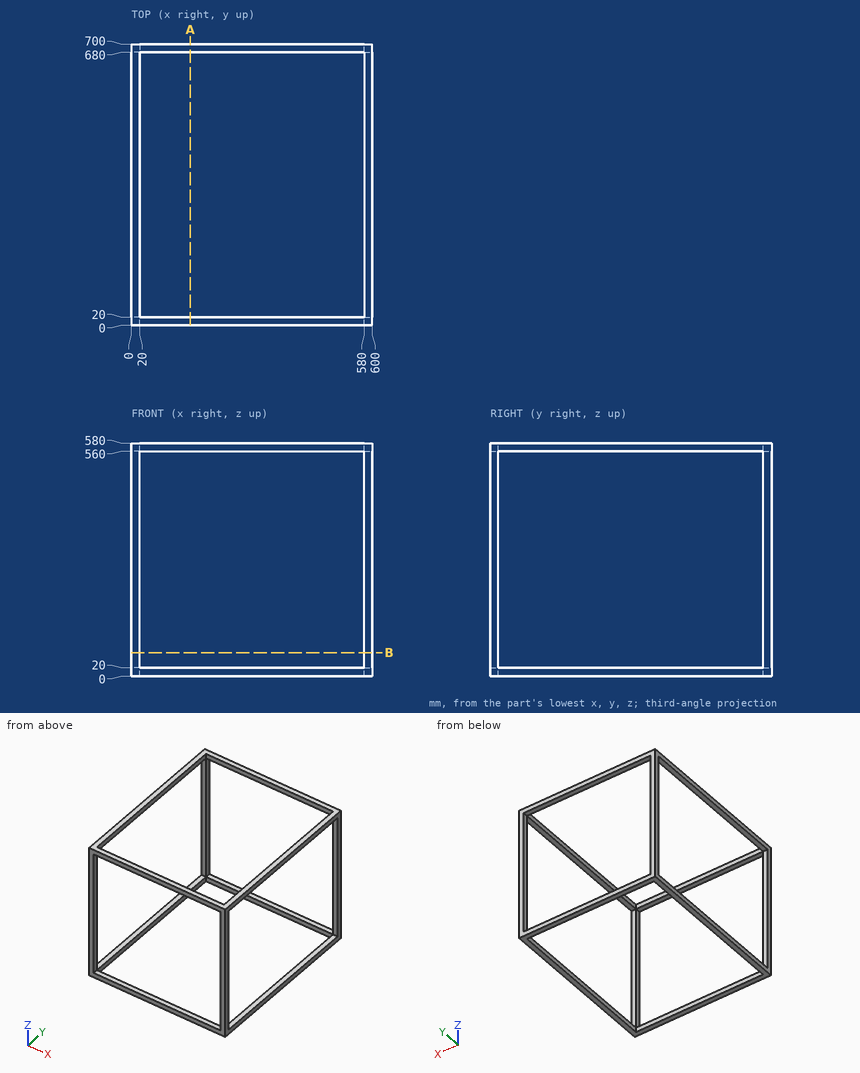
Source: three-view drawing plus pictorial views. Frame: mm from the lowest corner of the part. Give positions to 0.01 mm unless a question says otherwise; leave off trailing zeros. Write each loop counter-clockwise with the first axis right and the second up, starting at its lowest first coordinate (ties: lowest second). Pieces come first, ordered by that corner, then holes. Notation, with made-up numbers: (-23.75, 30) -> (22.25, 30) arc R34 cw to (22.25, 60) -> close; hole circle Ø3 at (87.5, -19.75). An arc over 180 degrees is marked (long way). Write item = value, one per line.
Q1. Cut plane A-A on x = 146.5. Return loops of the section in (y, z), then the cut area to 3 significant figures.
Here are the results:
outline = (0, 0) -> (20, 0) -> (20, 20) -> (0, 20) -> close; (0, 560) -> (20, 560) -> (20, 580) -> (0, 580) -> close; (680, 0) -> (700, 0) -> (700, 20) -> (680, 20) -> close; (680, 560) -> (700, 560) -> (700, 580) -> (680, 580) -> close
area = 1,600 mm²
Q2. Cut plane B-B on z = 58.5. Return loops of the section in (x, y), then the cut area to 3 significant figures.
Here are the results:
outline = (0, 0) -> (20, 0) -> (20, 20) -> (0, 20) -> close; (0, 680) -> (20, 680) -> (20, 700) -> (0, 700) -> close; (580, 0) -> (600, 0) -> (600, 20) -> (580, 20) -> close; (580, 680) -> (600, 680) -> (600, 700) -> (580, 700) -> close
area = 1,600 mm²
Q3. First-contact query: pin 1 (16 mm diameter, centred on x = 587.5, z = 363, fed in from -Y). Flat tip, straight axial feed; report the tip coordinate or a pass-through.
Here are the results:
pin_1 = 0
